For this review, take the finished solid that the model builds, in its own axes (mm). A direction names the side the tool comes from. Give positions to 0.01 mm unless a question says otherwise; leave off trailing zeros. Write each loop counter-clockwise with the first axis right and the second up, starting at its lowest first coordinate (ties: lowest second). Pieces come first, ordered by that corner, then holes. Notation, with made-up numbers: M -32,38.5 L 18,38.5 A9 ccw 18,51.5 Z; hole C -27.75,8.5 d10. An arc over 180 degrees is marked long. Use one line per item in the form item = value. Start each with the question number.
Q1. Clearance check with a flat-ended pin moving along its axis: pin 1 Ø4.5 at (x, z) = (-7683.21, 7.5) entering from +Y. State where the tip first meets the part, or that it passes through.
Q2. Consider section C-C on z = 4.5. Write out the cut boundary in (x, y), and give its area (3 significant figures).
Q3. Consider section B-B on z = 7.5. Write out the cut boundary in (x, y), and give its area (3 significant figures).
Q4. Mouldability with a two-part tool opening along X and no side actions: class faces 1 (the flat face through (-7695.709, 2871, 7)), 2 (the flat face through (-7693, 2880.865, 7)), 3 (the cylindrical face through (-7684.957, 2863.33, 7.577)), 4 (the cylindrical face through (-7690.41, 2866.15, 7.6)) as released by +X, released by -X, zero draft, split by the parting line, or undercut.
Q5. Consider section A-A on x = -7692.75. Write out the cut boundary in (y, z).
Q6. Tool access review of faces 5 (the flat face through (-7675.709, 2863, 7)), 6 (the flat face through (-7681, 2865.865, 7)): name each direction out of +Z, -Z, +X, -X, +Y, -Y from which nothing blocks a thin tool from reaching the whole face with its end or side.
Q7. For probe 1 along X at (y, z) = (2879.25, 10.25); probe 2 along Z at (x, y) = (-7682.75, 2865.5); probe 3 along Y at (x, z) = (-7686, 13.25), list the stretches that pass through material, from the lowest coordinate up. Write a range as [from, to].
Q8. Consider section D-D on y = 2877. Write out the cut boundary in (x, z).
```python
from build123d import *

# Parameters (mm, degrees)
F0_W     = 15
F0_H     = 5
F1_DEPTH = 15
F3_R     = 1.5
F4_DEPTH = 127
F5_D     = 3.5
F6_R     = 2
F7_R     = 2
F8_R     = 1


with BuildPart() as f1:
    # F0 (on Top) → F1 (new body)
    with BuildSketch(Plane.XY):
        Polygon((-7695.709171, 2880.865144), (-7695.709171, 2860.865144), (-7690.709171, 2860.865144), (-7690.709171, 2865.865144), (-7690.709171, 2880.865144), align=None)
        with Locations((-7683.209171, 2863.365144)):
            Rectangle(F0_W, F0_H)
    extrude(amount=F1_DEPTH)

    # F3 (on face) → F4 (cut)
    with BuildSketch(Plane.YZ.offset(-7690.709171)):
        with Locations((2873.365144, 7.5)):
            Circle(F3_R)
    extrude(amount=-F4_DEPTH, mode=Mode.SUBTRACT)

    # F5 (through all)
    with Locations(Plane(origin=(0, 2865.865144, 0), x_dir=(-1, 0, 0), z_dir=(0, 1, 0))):
        with Locations((7683.209171, 7.5)):
            Hole(F5_D / 2)

    # F6
    f6_edges = [f1.edges().sort_by_distance(p)[0] for p in [
        (-7693.209171, 2880.865144, 15),
        (-7693.209171, 2880.865144, 0),
    ]]
    fillet(f6_edges, radius=F6_R)

    # F7
    f7_edges = [f1.edges().sort_by_distance(p)[0] for p in [
        (-7675.709171, 2863.365144, 15),
        (-7675.709171, 2863.365144, 0),
    ]]
    fillet(f7_edges, radius=F7_R)

    # F8
    f8_edges = [f1.edges().sort_by_distance(p)[0] for p in [
        (-7690.709171, 2865.865144, 7.5),
    ]]
    fillet(f8_edges, radius=F8_R)


solid = f1.part
```
Working result:
q1.pin_1 = 2865.87
q2.outline = M -7695.71,2860.87 L -7675.71,2860.87 L -7675.71,2865.87 L -7689.71,2865.87 A1 cw -7690.71,2866.87 L -7690.71,2880.87 L -7695.71,2880.87 Z
q2.area = 175 mm²
q3.outline = M -7695.71,2860.87 L -7684.96,2860.87 L -7684.96,2865.87 L -7689.71,2865.87 A1 cw -7690.71,2866.87 L -7690.71,2871.87 L -7695.71,2871.87 Z; M -7695.71,2874.87 L -7690.71,2874.87 L -7690.71,2880.87 L -7695.71,2880.87 Z; M -7681.46,2860.87 L -7675.71,2860.87 L -7675.71,2865.87 L -7681.46,2865.87 Z
q3.area = 143 mm²
q4.face_1 = released by -X
q4.face_2 = zero draft
q4.face_3 = undercut
q4.face_4 = released by +X
q5.outline = M 2860.87,0 L 2878.87,0 A2 ccw 2880.87,2 L 2880.87,13 A2 ccw 2878.87,15 L 2860.87,15 Z; hole C 2873.37,7.5 d3
q6.face_5 = +Z, -Z, +X, +Y, -Y
q6.face_6 = +Z, -Z, +X, +Y
q7.probe_1 = [-7695.71, -7690.71]
q7.probe_2 = [0, 5.81], [9.19, 15]
q7.probe_3 = [2860.87, 2865.87]
q8.outline = M -7695.71,0 L -7690.71,0 L -7690.71,15 L -7695.71,15 Z
